Check sheet for the modelled part. Datum: model origin and axes. Units: mm. A direction names the side the tool comes from. Coordinates: 2 decimals unless noted, no trailing zeros. Write each loop counter-clockwise with the first axis right and the second up, starting at its lowest first coordinate (ties: lowest second). Pieces come first, ordered by that corner, then holes. Notation, with made-up numbers: (44.25, 43) - (48.25, 43) arc R35 cw to (48.25, 81) - close; hole circle Ø8 at (80.5, -23). An arc over 180 degrees is marked (long way). Use one line per item in the form item = value. Start each with the question number.
1. Cross-section at B-B on x = 52. Record the boundary of the cut face in (y, z), then the cut area to 3 significant figures.
2. Cross-section at A-A on z = 3. Record the boundary of the cut face in (x, y).
3. Tool access check on faces 1 (the face through (10.228, -4.7, -1.3)), 2 (the face through (0, -10, 84.9)), 3 (the face through (15, 3, 110)). Record the directions out of +Z, -Z, +X, -X, +Y, -Y that give a thin tool (end or side, any length) a straight path to the whole face; none if there is none.
4. Draft check along Y on faces 4 (the face through (0, -9.25, 39)), 5 (the face through (0, -12.25, -90)), 6 (the face through (15, 3, -110)). Enter one of: +Y half, -Y half, draft (parallel to the pull), parting line (faces both ways), or undercut.
5. Cross-section at C-C on z = 72. Record the boundary of the cut face in (x, y), then the cut area to 3 significant figures.
6. Go/stop test with flat-tipped pins: pin 1 Ø1.5 at (y, z) = (2.5, 109.5) entering from -X; pin 2 Ø1.5 at (x, y) = (-9, -7) entering from +Z; pin 3 Ø8 at (y, z) = (-6.5, 87) entering from -X. Record where each tip stops, or that it passes through.
7. Scan lines: line 1 along X through (y, z) = (-8.25, -93.5); line 2 along Y through (x, z) = (21.5, 95); line 3 along Z through (x, y) = (-7, -4.25). Record each from-to range of solid material in increasing order.
```python
from build123d import *

# Parameters (mm, degrees)
SZKIC1_W                        = 230
SZKIC1_H                        = 230
DODANIE_WYCI_GNI_CIE1_DEPTH     = 5
WYTNIJ_WYCI_GNI_CIE1_DEPTH      = 163.711400953
ZAOKR_GLENIE2_R                 = 5
SZYK_KO_OWY1_COUNT              = 4
ZAOKR_GLENIE2_OF_SZYK_KO_OWY1_R = 5
SZKIC3_W                        = 30
SZKIC3_H                        = 10
WYTNIJ_WYCI_GNI_CIE2_DEPTH      = 163.711400953
SZKIC4_W                        = 20.455701668
SZKIC4_H                        = 190
DODANIE_WYCI_GNI_CIE2_DEPTH     = 5
SZKIC5_W                        = 3
SZKIC5_H                        = 10
DODANIE_WYCI_GNI_CIE3_DEPTH     = 4.25
SZKIC6_W                        = 20.455701668
SZKIC6_H                        = 10.031438373
DODANIE_WYCI_GNI_CIE4_DEPTH     = 3
SZYK_LINIOWY1_COUNT             = 8
SZYK_LINIOWY1_PITCH             = 25.7


with BuildPart() as part:
    # Szkic1 → Dodanie-wyciągnięcie1 (new body)
    with BuildSketch(Plane(origin=(0, 0, 0), x_dir=(1, 0, 0), z_dir=(0, 1, 0))):
        Rectangle(SZKIC1_W, SZKIC1_H)
    extrude(amount=DODANIE_WYCI_GNI_CIE1_DEPTH)

    # Szkic2 → Wytnij-wyciągnięcie1 (cut, symmetric)
    with BuildSketch(Plane(origin=(0, 5, 0), x_dir=(1, 0, 0), z_dir=(0, 1, 0))):
        Polygon((-115, 115), (-64.088311755, 115), (-82.473088065, 96.615223689), (-89.544155877, 103.686291501), (-103.686291501, 89.544155877), (-96.615223689, 82.473088065), (-115, 64.088311755), align=None)
    wytnij_wyci_gni_cie1 = extrude(amount=WYTNIJ_WYCI_GNI_CIE1_DEPTH, both=True, mode=Mode.SUBTRACT)

    # Zaokrąglenie2
    zaokr_glenie2_edges = [part.edges().sort_by_distance(p)[0] for p in [
        (-82.473088065, 2.5, -96.615223689),
        (-96.615223689, 2.5, -82.473088065),
    ]]
    fillet(zaokr_glenie2_edges, radius=ZAOKR_GLENIE2_R)
    zaokr_glenie2_2_edges = [part.edges().sort_by_distance(p)[0] for p in [
        (-89.544155877, 2.5, -103.686291501),
        (-103.686291501, 2.5, -89.544155877),
    ]]
    fillet(zaokr_glenie2_2_edges, radius=ZAOKR_GLENIE2_R - 0.0001)  # a hair under: the kernel refuses the full size

    # Szyk kołowy1: Wytnij-wyciągnięcie1 ×4 about axis
    szyk_ko_owy1_axis = Axis((0, 0, 0), (0, 1, 0))
    for i in range(1, SZYK_KO_OWY1_COUNT):
        add(wytnij_wyci_gni_cie1.rotate(szyk_ko_owy1_axis, i * 360 / SZYK_KO_OWY1_COUNT), mode=Mode.SUBTRACT)

    # Zaokrąglenie2 of Szyk kołowy1
    zaokr_glenie2_of_szyk_ko_owy1_edges = [part.edges().sort_by_distance(p)[0] for p in [
        (-96.615223689, 2.5, 82.473088065),
        (-82.473088065, 2.5, 96.615223689),
        (82.473088065, 2.5, 96.615223689),
        (96.615223689, 2.5, 82.473088065),
        (96.615223689, 2.5, -82.473088065),
        (82.473088065, 2.5, -96.615223689),
    ]]
    fillet(zaokr_glenie2_of_szyk_ko_owy1_edges, radius=ZAOKR_GLENIE2_OF_SZYK_KO_OWY1_R)
    zaokr_glenie2_of_szyk_ko_owy1_2_edges = [part.edges().sort_by_distance(p)[0] for p in [
        (-103.686291501, 2.5, 89.544155877),
        (-89.544155877, 2.5, 103.686291501),
        (89.544155877, 2.5, 103.686291501),
        (103.686291501, 2.5, 89.544155877),
        (103.686291501, 2.5, -89.544155877),
        (89.544155877, 2.5, -103.686291501),
    ]]
    fillet(zaokr_glenie2_of_szyk_ko_owy1_2_edges, radius=ZAOKR_GLENIE2_OF_SZYK_KO_OWY1_R - 0.0001)  # a hair under: the kernel refuses the full size

    # Szkic3 → Wytnij-wyciągnięcie2 (cut, through all)
    with BuildSketch(Plane(origin=(0, 5, 0), x_dir=(1, 0, 0), z_dir=(0, 1, 0))):
        with Locations((0, -110)):
            Rectangle(SZKIC3_W, SZKIC3_H)
    wytnij_wyci_gni_cie2 = extrude(amount=-WYTNIJ_WYCI_GNI_CIE2_DEPTH, mode=Mode.SUBTRACT)

    # Lustro1: Wytnij-wyciągnięcie2 across plane
    add(wytnij_wyci_gni_cie2.mirror(Plane.XY), mode=Mode.SUBTRACT)

    # Szkic4 → Dodanie-wyciągnięcie2 (add)
    with BuildSketch(Plane.XZ):
        Rectangle(SZKIC4_W, SZKIC4_H)
    extrude(amount=DODANIE_WYCI_GNI_CIE2_DEPTH)

    # Szkic5 → Dodanie-wyciągnięcie3 (add)
    with BuildSketch(Plane.XZ.offset(5)):
        with Locations((8.727850834, -90)):
            Rectangle(SZKIC5_W, SZKIC5_H)
        with Locations((-8.727850834, -90)):
            Rectangle(SZKIC5_W, SZKIC5_H)
    dodanie_wyci_gni_cie3 = extrude(amount=DODANIE_WYCI_GNI_CIE3_DEPTH)

    # Szkic6 → Dodanie-wyciągnięcie4 (add)
    with BuildSketch(Plane.XZ.offset(9.25)):
        with Locations((0, -89.984280813)):
            Rectangle(SZKIC6_W, SZKIC6_H)
    dodanie_wyci_gni_cie4 = extrude(amount=DODANIE_WYCI_GNI_CIE4_DEPTH)

    # Szyk liniowy1: Dodanie-wyciągnięcie3, Dodanie-wyciągnięcie4 ×8
    with Locations(*[(0, 0, i * SZYK_LINIOWY1_PITCH) for i in range(1, SZYK_LINIOWY1_COUNT)]):
        add(dodanie_wyci_gni_cie3)
        add(dodanie_wyci_gni_cie4)


solid = part.part
```
Final values:
q1.outline = (0, -115) - (5, -115) - (5, 115) - (0, 115) - close
q1.area = 1,150 mm²
q2.outline = (-115, 0) - (-10.23, 0) - (-10.23, -5) - (10.23, -5) - (10.23, 0) - (115, 0) - (115, 5) - (-115, 5) - close
q3.face_1 = +Z, -Z, +X, -Y
q3.face_2 = +X, -X, -Y
q3.face_3 = +Z, +Y, -Y
q4.face_4 = undercut
q4.face_5 = -Y half
q4.face_6 = draft
q5.outline = (-107.09, 0) - (-10.23, 0) - (-10.23, -5) - (10.23, -5) - (10.23, 0) - (107.09, 0) - (107.09, 5) - (-107.09, 5) - close
q5.area = 1,170 mm²
q6.pin_1 = -70.34
q6.pin_2 = 94.9
q6.pin_3 = -10.23
q7.line_1 = -10.23 to -7.23, 7.23 to 10.23
q7.line_2 = 0 to 5
q7.line_3 = -95 to 95
